from build123d import *

# Parameters (mm, degrees)
F0_W     = 100
F0_H     = 60
F1_DEPTH = 5
F2_R     = 5
F3_DEPTH = 25
F5_DEPTH = 22


with BuildPart() as f1:
    # F0 (on Top) → F1 (new body)
    with BuildSketch(Plane.XY):
        Rectangle(F0_W, F0_H)
    extrude(amount=F1_DEPTH)

    # F2 (on face) → F3 (cut)
    with BuildSketch(Plane.XY.offset(5)):
        with Locations((37.62725, 19.000012)):
            Circle(F2_R)
    extrude(amount=-F3_DEPTH, mode=Mode.SUBTRACT)

    # F4 (on face) → F5 (join)
    with BuildSketch(Plane.XY.offset(5)):
        Polygon((-13.507203, 3.325971), (-16.744654, 11.239743), (-24.950408, 13.642757), (-31.945364, 8.725496), (-32.462178, 0.190757), (-26.111678, -5.534628), (-17.675921, -4.139326), align=None)
    extrude(amount=F5_DEPTH)


solid = f1.part
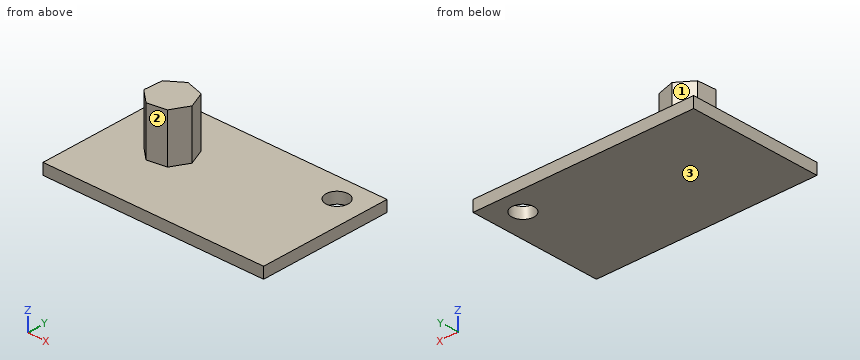
The model under review builds one solid part; all positions refer to its coordinate system, in mm. Face numbers are marked on the shaded views. A direction names the side the tool comes from. Round coordinates to 2 decimals unless told otherwise and drop trailing zeros. Order: outer loops, then holes, each group sorted by start corner. A loop starts at its lowest first (then second) coordinate and runs counter-clockwise, first axis right, second up. Notation, with made-up numbers: (84, 72) -> (121, 72) arc R27 cw to (121, 108) -> close; hole circle Ø8 at (82.25, 0). An arc over 180 degrees is marked (long way). Write item = value, one per line. Start each with the question number.
Item 1: Consider section C-C on x = -15. Write out the cut boundary in (y, z).
Item 2: For the marked faces 1, 2 and 3, list the 3-axis set-ups (+Z, -Z, +X, -X, +Y, -Y) from which the entire face can be reached by the end or side of a thin tool; tool diameter is ignored.
Item 3: Consider section D-D on y = -16. Write out the cut boundary in (x, z).
Item 4: Consider section A-A on y = 18. Write out the cut boundary in (x, z), plus the area to 3 significant figures.
Item 5: Consider section B-B on z = 16. Write out the cut boundary in (x, y), plus the area to 3 significant figures.
Item 6: For line 1 along Z through (x, y) = (9, 3); line 2 along Y through (x, z) = (-31, 13); line 3 along X through (y, z) = (7.5, 16.5), list the stretches that pass through material, from the lowest coordinate up.
Item 7: Clearance check with flat-ended pins moving along their axes: pin 1 Ø2 at (y, z) = (-2.5, 9.5) entering from +X; pin 2 Ø6 at (x, z) = (-35, 22.5) entering from -Y. State where each tip first meets the part, or that it passes through.
Conclusion:
q1.outline = (-30, 0) -> (30, 0) -> (30, 5) -> (6.98, 5) -> (6.98, 27) -> (0.65, 27) -> (0.65, 5) -> (-30, 5) -> close
q2.face_1 = +Z, -X, +Y
q2.face_2 = +Z, +X, -Y
q2.face_3 = -Z, +X, -X, +Y, -Y
q3.outline = (-50, 0) -> (50, 0) -> (50, 5) -> (-50, 5) -> close
q4.outline = (-50, 0) -> (32.73, 0) -> (32.73, 5) -> (-50, 5) -> close; (42.53, 0) -> (50, 0) -> (50, 5) -> (42.53, 5) -> close
q4.area = 451 mm2
q5.outline = (-32.46, 0.19) -> (-26.11, -5.53) -> (-17.68, -4.14) -> (-13.51, 3.33) -> (-16.74, 11.24) -> (-24.95, 13.64) -> (-31.95, 8.73) -> close
q5.area = 266 mm2
q6.line_1 = 0 to 5
q6.line_2 = -1.13 to 9.39
q6.line_3 = -32.02 to -15.21
q7.pin_1 = -16.2
q7.pin_2 = -0.23
